Could you check a few things on this model? Use its own coordinates, in mm. Face numbers are marked on the shaded views. A direction names the side the tool comes from. Coordinates: 2 decimals unless noted, no trailing zeros. Write each loop counter-clockwise with the first axis right and the second up, starting at its lowest first coordinate (ties: lowest second). Pieces come first, ordered by that corner, then holes.
Item 1: I want a section at C-C on z = 4. Please give me the cut outline in (x, y).
Item 2: I want a section at B-B on y = 19. Please give me the cut outline in (x, z), then the cut area to 3 significant figures.
Item 3: If I drill on probe 1 along Z at (x, y) = (7, 53); probe 2 along Z at (x, y) = (7, 53.1); probe 3 along Y at (x, z) = (-2, -14), over which ranges is the centre line in solid material (lowest first)?
Item 4: I want a section at D-D on x = -12. Please give me the cut outline in (y, z).
Item 5: Which directions (+Z, -Z, +X, -X, +Y, -Y) give clear straight access to the entire face, cutting with the end or side of a thin tool? Please do the marked faces 1 and 2.
Item 6: I want a section at A-A on x = 0. Please give me the cut outline in (y, z), then the cut area to 3 significant figures.
Item 7: For P1, Ø3, axis at x = -10, y = 25.5, coming from the -Z side; P2, Ø2, axis at x = 7, z = 12.12, coming from the +Y side; P3, Ø6, axis at x = -15, y = 47, coming from the +Z side, each with a flat end and sliding along its axis, tell me the tip position at first contact or that it passes through.
from build123d import *

# Parameters (mm, degrees)
M3_TAPPED_HOLE1_D     = 2.5
M3_TAPPED_HOLE1_DEPTH = 0.16
M3_TAPPED_HOLE1_TIP   = 0.751075774


with BuildPart() as part:
    # Sketch1 → Revolve1 (revolve)
    with BuildSketch(Plane(origin=(0, 0, 0), x_dir=(0, 0, -1), z_dir=(1, 0, 0)), mode=Mode.PRIVATE) as revolve1_sk:
        Polygon((0, 0), (19.2, 0), (19.2, 53.2), (7.5, 53.2), (7.5, 56.7), (2.5, 56.7), (2.5, 73.7), (0, 73.7), align=None)
    revolve(revolve1_sk.sketch.rotate(Axis((0, 33.970588235, 0), (0, -1, 0)), 180), axis=Axis((0, 33.970588235, 0), (0, -1, 0)))

    # M3 Tapped Hole1
    with Locations(Plane(origin=(0, 53.2, 0), x_dir=(1, 0, 0), z_dir=(0, 1, 0))):
        with Locations((7, 12.124355653), (7, -12.124355653), (-14, 0)):
            Hole(M3_TAPPED_HOLE1_D / 2, depth=M3_TAPPED_HOLE1_DEPTH)
            with Locations((0, 0, -(M3_TAPPED_HOLE1_DEPTH + M3_TAPPED_HOLE1_TIP / 2))):  # 118° drill point
                Cone(0, M3_TAPPED_HOLE1_D / 2, M3_TAPPED_HOLE1_TIP, mode=Mode.SUBTRACT)


solid = part.part
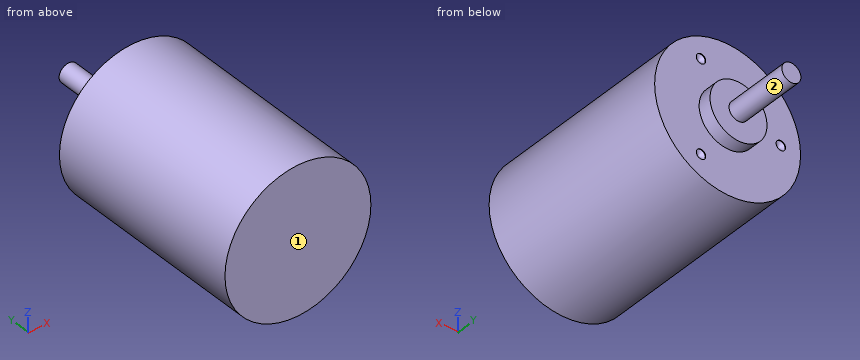
Response values:
1. outline: (-18.78, 0) - (18.78, 0) - (18.78, 53.2) - (6.34, 53.2) - (6.34, 56.7) - (-6.34, 56.7) - (-6.34, 53.2) - (-18.78, 53.2) - close
2. outline: circle Ø38.4 at (0, 0)
2. area: 1,160 mm2
3. probe 1: z = -17.88 to -13.31, -10.94 to 10.94, 13.31 to 17.88
3. probe 2: z = -17.88 to -13.37, -10.87 to 10.87, 13.37 to 17.88
3. probe 3: y = 0 to 53.2
4. outline: (0, -14.99) - (53.2, -14.99) - (53.2, 14.99) - (0, 14.99) - close
5. face 1: +Z, -Z, +X, -X, -Y
5. face 2: +Y
6. outline: (0, -19.2) - (53.2, -19.2) - (53.2, -7.5) - (56.7, -7.5) - (56.7, -2.5) - (73.7, -2.5) - (73.7, 2.5) - (56.7, 2.5) - (56.7, 7.5) - (53.2, 7.5) - (53.2, 19.2) - (0, 19.2) - close
6. area: 2,180 mm2
7. P1: stops at z = -17.22
7. P2: stops at y = 52.89
7. P3: stops at z = 14.99
